from build123d import *

# Parameters (mm, degrees)
F1_DEPTH = 12
F3_W     = 2.5
F3_H     = 12
F4_DEPTH = 9.464
F5_R     = 0.5


with BuildPart() as f1:
    # F0 (on Top) → F1 (new body)
    with BuildSketch(Plane.XY):
        Polygon((-13.856406, 0), (0, 0), (-3.464102, 6), align=None)
    extrude(amount=F1_DEPTH)

    # F3 (on offset) → F4 (join)
    with BuildSketch(Plane.YZ.offset(-3.4643)):
        with Locations((1.25, 6)):
            Rectangle(F3_W, F3_H)
    extrude(amount=F4_DEPTH)

    # F5
    f5_edges = [f1.edges().sort_by_distance(p)[0] for p in [
        (-3.464102, 6, 6),
        (-13.856406, 0, 6),
    ]]
    fillet(f5_edges, radius=F5_R)


solid = f1.part
Read the model definition and answer for the solid it produces. Units are mm, in the model's axes. A direction names the side the tool comes from. Give positions to 0.01 mm unless a question says otherwise; leave off trailing zeros. Write each loop counter-clockwise with the first axis right and the second up, starting at its lowest first coordinate (ties: lowest second). Pieces come first, ordered by that corner, then holes. Notation, with made-up numbers: (-29.5, 10) -> (22.5, 10) arc R23 ccw to (22.5, 44) -> close; hole circle Ø1 at (51, -36). An arc over 180 degrees is marked (long way). Answer as a JSON object with one key per item and string values. Group by question number.
1) A tool of negligible diameter and unlimited length cuts with its end or side. For faces 1 (the flat face through (2, 2.5, 6)), 2 (the flat face through (-3, 2, 12)), from which of +Z, -Z, +X, -X, +Y, -Y can it reach the whole face along a straight path? Write none if from no direction.
2) Each of these flat-tipped pins is pushed along its axis until it touches: P1, Ø3, axis at y = 1, z = 3.5, coming from the -X side; P2, Ø3.5, axis at x = 1.5, z = 6.5, coming from the +Y side. Where does it stop, or does it pass through?
3) Find section A-A (z = 2.5). Write down the section's boundary in (x, y), and give its area (3 significant figures).
4) Find section C-C (y = 4.8). Write down the section's boundary in (x, z), and give its area (3 significant figures).
5) Consider L1, parallel to Y at x = 2.25, z = 1; L2, parallel to X at y = 5.15, z = 3.25; L3, parallel to Y at x = -9, z = 3.25. Determine where each line is inside the solid, lowest interval first. Write a range as from..to.
6) Find section B-B (x = 2.75). Write down the section's boundary in (y, z).
Values follow:
{
 "1": {"face 1": "+Z, -Z, +X, +Y", "face 2": "+Z, +X, -X, +Y, -Y"},
 "2": {"P1": "stops at x = -12.49", "P2": "stops at y = 2.5"},
 "3": {"outline": "(-12.24, 0.93) arc R0.5 ccw to (-11.99, 0) -> (6, 0) -> (6, 2.5) -> (-1.44, 2.5) -> (-3.21, 5.57) arc R0.5 ccw to (-3.9, 5.75) -> close", "area": "57.7 mm2"},
 "4": {"outline": "(-5.54, 0) -> (-2.77, 0) -> (-2.77, 12) -> (-5.54, 12) -> close", "area": "33.3 mm2"},
 "5": {"L1": "y = 0..2.5", "L2": "x = -4.94..-2.97", "L3": "y = 0..2.8"},
 "6": {"outline": "(0, 0) -> (2.5, 0) -> (2.5, 12) -> (0, 12) -> close"}
}
